from build123d import *

# Parameters (mm, degrees)
F0_W     = 38.1
F0_H     = 279.4
F1_DEPTH = 6.35
F2_W     = 25.4
F2_H     = 6.35
F4_DEPTH = 6.35
F3_W     = 25.4
F3_H     = 6.35
F5_DEPTH = 6.35
F6_W     = 25.4
F6_H     = 6.35
F7_DEPTH = 6.35


with BuildPart() as f1:
    # F0 (on Top) → F1 (new body)
    with BuildSketch(Plane.XY):
        with Locations((19.05, 139.7)):
            Rectangle(F0_W, F0_H)
    extrude(amount=F1_DEPTH)

    # F2 (on face) → F4 (join)
    with BuildSketch(Plane.YZ.offset(38.1)):
        with Locations((241.3, 3.175)):
            Rectangle(F2_W, F2_H)
        with Locations((190.5, 3.175)):
            Rectangle(F2_W, F2_H)
        with Locations((139.7, 3.175)):
            Rectangle(F2_W, F2_H)
        with Locations((88.9, 3.175)):
            Rectangle(F2_W, F2_H)
        with Locations((38.1, 3.175)):
            Rectangle(F2_W, F2_H)
    extrude(amount=F4_DEPTH)

    # F3 (on face) → F5 (join)
    with BuildSketch(Plane(origin=(0, 0, 0), x_dir=(0, -1, 0), z_dir=(-1, 0, 0))):
        with Locations((-38.1, 3.175)):
            Rectangle(F3_W, F3_H)
        with Locations((-88.9, 3.175)):
            Rectangle(F3_W, F3_H)
        with Locations((-139.7, 3.175)):
            Rectangle(F3_W, F3_H)
        with Locations((-190.5, 3.175)):
            Rectangle(F3_W, F3_H)
        with Locations((-241.3, 3.175)):
            Rectangle(F3_W, F3_H)
    extrude(amount=F5_DEPTH)

    # F6 (on face) → F7 (cut)
    with BuildSketch(Plane(origin=(0, 279.4, 0), x_dir=(-1, 0, 0), z_dir=(0, 1, 0))):
        with Locations((-19.05, 3.175)):
            Rectangle(F6_W, F6_H)
    extrude(amount=-F7_DEPTH, mode=Mode.SUBTRACT)


solid = f1.part
Read the model definition and answer for the solid it produces. Units are mm, in the model's axes. A direction names the side the tool comes from. Round coordinates to 2 decimals unless told otherwise and drop trailing zeros. Write each loop counter-clockwise with the first axis right and the second up, starting at its lowest first coordinate (ties: lowest second). Pieces come first, ordered by that corner, then holes.
Q1. The mould has two halves that part along Y. Classify faces 6 (the face through (41, 50.8, 3)), 7 (the face through (-3, 152.4, 3)), 8 (the face through (19, 273.05, 3)), 9 (the face through (41, 25.4, 3)): released by +Y, released by -Y, zero draft, split by the parting line, or undercut.
Values:
face 6: undercut
face 7: undercut
face 8: released by +Y
face 9: released by -Y
Q2. Find section B-B on y = 169. Determine the outline of the cut face in (x, z).
Values:
outline: (0, 0) - (38.1, 0) - (38.1, 6.35) - (0, 6.35) - close
Q3. Flat-ended cylindrical pins translate along their axes: P1, Ø3, axis at x = -4, z = 3, coming from the +Y side; P2, Ø1.9, axis at y = 169, z = 3.5, coming from the +X side; P3, Ø3, axis at x = -2, z = 2.5, coming from the -Y side. Find the tip coordinate at first contact, or state that the pin passes through.
Values:
P1: stops at y = 254
P2: stops at x = 38.1
P3: stops at y = 25.4
Q4. Find section C-C on x = 16. Determine the outline of the cut face in (y, z), and give its area (3 significant figures).
Values:
outline: (0, 0) - (273.05, 0) - (273.05, 6.35) - (0, 6.35) - close
area: 1,730 mm2
Q5. Find section A-A on x = 41.5. Determine the outline of the cut face in (y, z).
Values:
outline: (25.4, 0) - (50.8, 0) - (50.8, 6.35) - (25.4, 6.35) - close; (76.2, 0) - (101.6, 0) - (101.6, 6.35) - (76.2, 6.35) - close; (127, 0) - (152.4, 0) - (152.4, 6.35) - (127, 6.35) - close; (177.8, 0) - (203.2, 0) - (203.2, 6.35) - (177.8, 6.35) - close; (228.6, 0) - (254, 0) - (254, 6.35) - (228.6, 6.35) - close
Q6. Straight lines are drawn through the part: line 1 (Y direction, x = 41, z = 4.25); line 2 (Y direction, x = 28.5, z = 4); line 3 (X direction, y = 158.5, z = 3.5). For each, find the intervals that lie inside material, in ascending order.
Values:
line 1: y = 25.4 to 50.8, 76.2 to 101.6, 127 to 152.4, 177.8 to 203.2, 228.6 to 254
line 2: y = 0 to 273.05
line 3: x = 0 to 38.1
Q7. A tool of negligible diameter and unlimited length cuts with its end or side. For faces 1 (the face through (41, 254, 3)), 2 (the face through (0, 63, 3)), 3 (the face through (31.75, 276, 3)), 4 (the face through (0, 13, 3)), 5 (the face through (41, 177.8, 3)), from which of +Z, -Z, +X, -X, +Y, -Y can it reach the whole face along a straight path? Write none if from no direction.
Values:
face 1: +Z, -Z, +X, +Y
face 2: +Z, -Z, -X
face 3: +Z, -Z, +Y
face 4: +Z, -Z, -X, -Y
face 5: +Z, -Z, +X
